from build123d import *

# Parameters (mm, degrees)
RESSALTO_EXTRUS_O1_DEPTH = 5
ESBO_O2_R                = 12.2
CORTE_EXTRUS_O1_DEPTH    = 6
FILETE1_R                = 1
ESBO_O3_W                = 27.5
ESBO_O3_H                = 5
ESBO_O3_W_2              = 65
CORTE_EXTRUS_O2_DEPTH    = 6
CORTE_EXTRUS_O3_DEPTH    = 6
ESBO_O5_R                = 1.5
ESBO_O5_R_2              = 1.036414637
CORTE_EXTRUS_O4_DEPTH    = 6
ESBO_O6_W                = 43.400181399
ESBO_O6_H                = 3
CORTE_EXTRUS_O5_DEPTH    = 6


with BuildPart() as part:
    # Esboço1 → Ressalto-extrusão1 (new body)
    with BuildSketch(Plane.XY):
        with BuildLine():
            Line((20, 0), (170, 0))
            ThreePointArc((170, 0), (184.142135624, 5.857864376), (190, 20))
            Line((190, 20), (190, 25))
            Line((190, 25), (0, 25))
            Line((0, 25), (0, 20))
            ThreePointArc((0, 20), (5.857864376, 5.857864376), (20, 0))
        make_face()
    extrude(amount=RESSALTO_EXTRUS_O1_DEPTH)

    # Esboço2 → Corte-extrusão1 (cut, through all)
    with BuildSketch(Plane(origin=(0, 0, 0), x_dir=(-1, 0, 0), z_dir=(0, 0, -1))):
        with Locations((-50, 2.8)):
            Circle(ESBO_O2_R)
        with Locations((-140, 2.8)):
            Circle(ESBO_O2_R)
    extrude(amount=-CORTE_EXTRUS_O1_DEPTH, mode=Mode.SUBTRACT)

    # Filete1
    filete1_edges = [part.edges().sort_by_distance(p)[0] for p in [
        (61.874342087, 0, 2.5),
        (38.125657913, 0, 2.5),
        (151.874342087, 0, 2.5),
        (128.125657913, 0, 2.5),
    ]]
    fillet(filete1_edges, radius=FILETE1_R)

    # Esboço3 → Corte-extrusão2 (cut, through all)
    with BuildSketch(Plane(origin=(0, 0, 0), x_dir=(-1, 0, 0), z_dir=(0, 0, -1))):
        with Locations((-166.25, 22.5)):
            Rectangle(ESBO_O3_W, ESBO_O3_H)
        with Locations((-95, 22.5)):
            Rectangle(ESBO_O3_W_2, ESBO_O3_H)
        with Locations((-23.75, 22.5)):
            Rectangle(ESBO_O3_W, ESBO_O3_H)
    extrude(amount=-CORTE_EXTRUS_O2_DEPTH, mode=Mode.SUBTRACT)

    # Esboço4 → Corte-extrusão3 (cut, through all)
    with BuildSketch(Plane(origin=(0, 0, 0), x_dir=(-1, 0, 0), z_dir=(0, 0, -1))):
        Polygon((-24.75, 13), (-24.75, 15), (-26.55, 15), (-26.55, 16.5), (-24.75, 16.5), (-24.75, 20), (-22.75, 20), (-22.75, 16.5), (-20.95, 16.5), (-20.95, 15), (-22.75, 15), (-22.75, 13), align=None)
        Polygon((-96, 13), (-96, 15), (-97.8, 15), (-97.8, 16.5), (-96, 16.5), (-96, 20), (-94, 20), (-94, 16.5), (-92.2, 16.5), (-92.2, 15), (-94, 15), (-94, 13), align=None)
        Polygon((-167.25, 13), (-167.25, 15), (-169.05, 15), (-169.05, 16.5), (-167.25, 16.5), (-167.25, 20), (-165.25, 20), (-165.25, 16.5), (-163.45, 16.5), (-163.45, 15), (-165.25, 15), (-165.25, 13), align=None)
    extrude(amount=-CORTE_EXTRUS_O3_DEPTH, mode=Mode.SUBTRACT)

    # Esboço5 → Corte-extrusão4 (cut, through all)
    with BuildSketch(Plane.XY.offset(5)):
        with Locations((180, 10)):
            Circle(ESBO_O5_R)
        with Locations((10, 10)):
            Circle(ESBO_O5_R)
        with Locations((15.588408084, 15.09127059)):
            Circle(ESBO_O5_R_2)
    extrude(amount=-CORTE_EXTRUS_O4_DEPTH, mode=Mode.SUBTRACT)

    # Esboço6 → Corte-extrusão5 (cut, through all)
    with BuildSketch(Plane.XY.offset(5)):
        Polygon((77.369700901, 6.5), (77.369700901, 3), (79.369700901, 3), (79.369700901, 6.5), (81.169700901, 6.5), (81.169700901, 8), (79.369700901, 8), (79.369700901, 10), (77.369700901, 10), (77.369700901, 8), (75.569700901, 8), (75.569700901, 6.5), align=None)
        with Locations((95.0697916, 1.5)):
            Rectangle(ESBO_O6_W, ESBO_O6_H)
        Polygon((110.7698823, 3), (112.7698823, 3), (112.7698823, 6.5), (114.5698823, 6.5), (114.5698823, 8), (112.7698823, 8), (112.7698823, 10), (110.7698823, 10), (110.7698823, 8), (108.9698823, 8), (108.9698823, 6.5), (110.7698823, 6.5), align=None)
    extrude(amount=-CORTE_EXTRUS_O5_DEPTH, mode=Mode.SUBTRACT)


solid = part.part
The model under review builds one solid part; all positions refer to its coordinate system, in mm. A direction names the side the tool comes from. Round coordinates to 2 decimals unless told otherwise and drop trailing zeros. Loops run counter-clockwise (first coordinate to the right, second up) from the corner with the lowest first, then second, coordinate; pieces in that order, holes last. Notation, with made-up numbers: M 19.5,-36 L 27.5,-36 A19 ccw 27.5,-4 Z; hole C -18,9.25 d10. An arc over 180 degrees is marked long. Answer as CSV lines item,"result". Start each with the question number.
Item 1: Consider section B-B (z = 2.6). State how many separate pieces and enclosed holes the cut face has, then the cut area to 3 significant figures.
Item 2: Consider section C-C (x = 84.5). Write out the cut boundary in (y, z).
Item 3: For faces 1 (the face through (24.75, 18, 2)), 2 (the face through (68, 0, 2)), 3 (the face through (115, 3, 3)), list the 3-axis set-ups (+Z, -Z, +X, -X, +Y, -Y) from which the entire face can be reached by the end or side of a thin tool; tool diameter is ignored.
Item 4: Consider section A-A (x = 50). Write out the cut boundary in (y, z), then the cut area to 3 significant figures.
Item 5: Mouldability with a two-part tool opening along Y and no side actions: class faces 4 (the face through (31, 20, 2)), 5 (the face through (112.77, 5, 3)), 6 (the face through (8.8, 9.1, 2.5)) as released by +Y, released by -Y, zero draft, split by the parting line, or undercut.
Item 6: Wall thickness on line 1 (X direction, y = 22, z = 4); line 2 (X direction, y = 2.8, z = 2.7); line 3 (Y direction, x = 109, z = 2.55): over which ranges is each line inside the solid? List them lowest first. Write a range as [from, to].
Item 7: Insertion check: P1, Ø3, axis at y = 10.5, z = 2, coming from the +X side; P2, Ø1, axis at x = 112, z = 2, coming from the -Y side; P3, Ø2, axis at x = 97, z = 1.5, coming from the +Y side. Each pin has a flat end and moves straight along its axis. Give the tip position at first contact, or say it passes through.
Answer:
1,separate pieces,"1"
1,enclosed holes,"3"
1,area,"3,130 mm^2"
2,outline,"M 3,0 L 20,0 L 20,5 L 3,5 Z"
3,face 1,"+Z, -Z, +Y"
3,face 2,"+Z, -Z, +X, -X, -Y"
3,face 3,"+Z, -Z, -Y"
4,outline,"M 15,0 L 25,0 L 25,5 L 15,5 Z"
4,area,"50.0 mm^2"
5,face 4,"released by +Y"
5,face 5,"zero draft"
5,face 6,"undercut"
6,line 1,"x = [0, 10], [37.5, 62.5], [127.5, 152.5], [180, 190]"
6,line 2,"x = [9.79, 37.8], [62.2, 73.37], [116.77, 127.8], [152.2, 180.21]"
6,line 3,"y = [3, 6.5], [8, 20]"
7,P1,"stops at x = 188.33"
7,P2,"stops at y = 10"
7,P3,"stops at y = 20"
